Geometry: see drawing. Coordinates: mm, zero at the bounding-box minimum. A direction names the side the tool comes from. Coordinates: 2 decimals unless noted, no trailing zeros. Order: outer loops, then holes, each group sorted by start corner. A loop starts at its lowest first (then second) coordinate and runs counter-clockwise, first axis right, second up. Notation, with made-up numbers: (50, 82) -> (104, 82) arc R18 ccw to (104, 106) -> close; hole circle Ø3 at (-13.75, 85). An arc over 180 degrees is marked (long way). One line per item, written item: value. Start each with the question number.
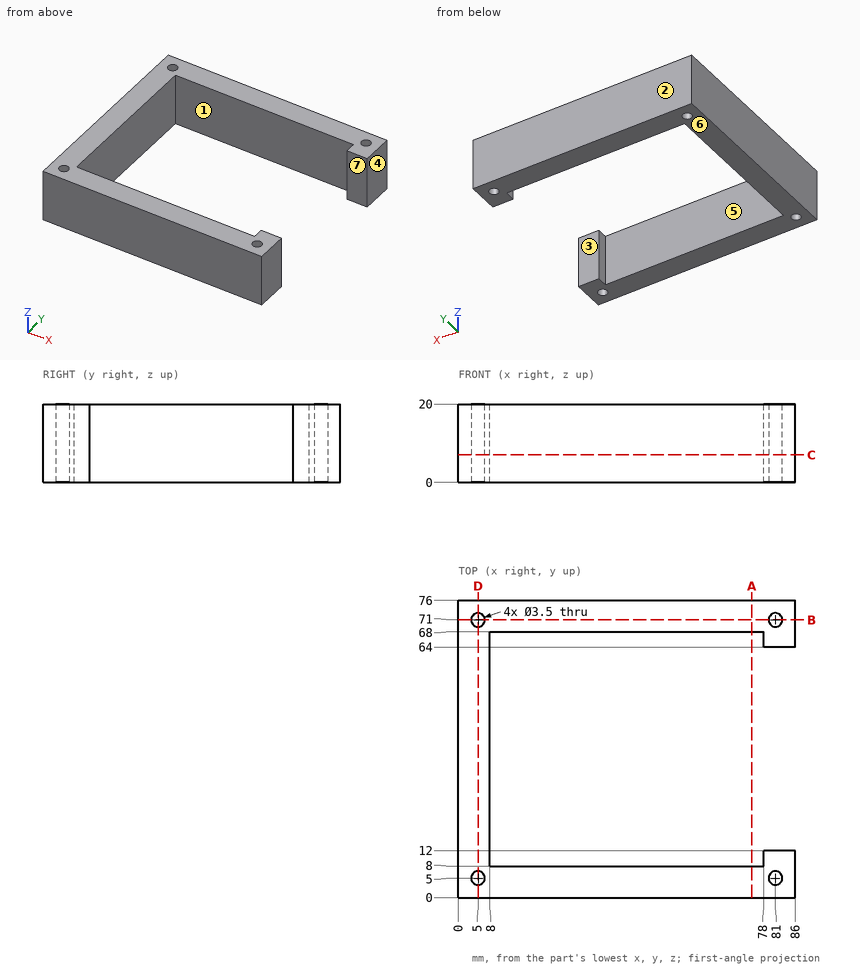
1) Section query D-D, the plane x = 5. Return the cut outline in (y, z).
2) Mould query, pull axis Y, two halves, no side actions, for the marked faces 1, 2, 3 and 4. Classes: +Y half, -Y half, draft (parallel to the pull), parting line (faces both ways), or undercut.
3) Access query for the marked faces 5, 6 and 7. Directions: +Z, -Z, +X, -X, +Y, -Y. A direction counts if a zero-diameter tool reaches every point of the face in a straight line with its end or side. Return the directions, or none.
4) Pin query (flat end, axial travel): pin 1 Ø3 at (x, y) = (81, 71) entering from +Z; pin 2 Ø1 at (y, z) = (62.5, 8.5) entering from -X; pin 3 Ø6 at (y, z) = (31.5, 9.5) entering from +X. Return the tip coordinate at first contact, or that it passes through.
5) Section query B-B, the plane y = 71. Return the cut outline in (x, z), plus the area to 3 significant figures.
6) Ray query, line 1 along Y through (x, z) = (5, 4); line 2 along X through (y, z) = (71, 5.25); line 3 along Y through (x, z) = (81, 4.5). Return the intervals inside material, ascending. Write a range as from..to.
7) Section query C-C, the plane z = 7. Return the cut outline in (x, y), plus the area to 3 significant figures.
8) Section query A-A, the plane x = 75. Return the cut outline in (y, z), plus the area to 3 significant figures.
Entries:
1. outline: (0, 0) -> (3.25, 0) -> (3.25, 20) -> (0, 20) -> close; (6.75, 0) -> (69.25, 0) -> (69.25, 20) -> (6.75, 20) -> close; (72.75, 0) -> (76, 0) -> (76, 20) -> (72.75, 20) -> close
2. face 1: undercut
2. face 2: +Y half
2. face 3: undercut
2. face 4: draft
3. face 5: +Z, -Z
3. face 6: -Z, +X, -X, +Y, -Y
3. face 7: +Z, -Z, +X
4. pin 1: passes through
4. pin 2: stops at x = 0
4. pin 3: stops at x = 8
5. outline: (0, 0) -> (3.25, 0) -> (3.25, 20) -> (0, 20) -> close; (6.75, 0) -> (79.25, 0) -> (79.25, 20) -> (6.75, 20) -> close; (82.75, 0) -> (86, 0) -> (86, 20) -> (82.75, 20) -> close
5. area: 1,580 mm2
6. line 1: y = 0..3.25, 6.75..69.25, 72.75..76
6. line 2: x = 0..3.25, 6.75..79.25, 82.75..86
6. line 3: y = 0..3.25, 6.75..12, 64..69.25, 72.75..76
7. outline: (0, 0) -> (86, 0) -> (86, 12) -> (78, 12) -> (78, 8) -> (8, 8) -> (8, 68) -> (78, 68) -> (78, 64) -> (86, 64) -> (86, 76) -> (0, 76) -> close; hole circle Ø3.5 at (5, 5); hole circle Ø3.5 at (5, 71); hole circle Ø3.5 at (81, 5); hole circle Ø3.5 at (81, 71)
7. area: 1,880 mm2
8. outline: (0, 0) -> (8, 0) -> (8, 20) -> (0, 20) -> close; (68, 0) -> (76, 0) -> (76, 20) -> (68, 20) -> close
8. area: 320 mm2
